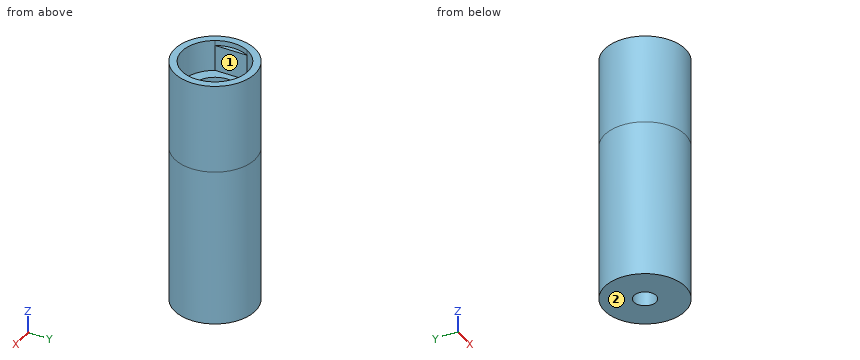
from build123d import *

# Parameters (mm, degrees)
F0_R     = 14.55
F1_DEPTH = 11.2
F2_DEPTH = 9.35
F0_R_2   = 7.975
F3_DEPTH = 21
F4_R     = 14.55
F4_R_2   = 4
F5_DEPTH = 57


with BuildPart() as f1:
    # F0 (on Top) → F1 (new body)
    with BuildSketch(Plane.XY):
        Circle(F0_R)
        with BuildLine():
            ThreePointArc((10.425, -5.7900777197), (0, -11.925), (-10.425, -5.7900777197))
            ThreePointArc((-10.425, -5.7900777197), (-11.925, 0), (-10.425, 5.7900777197))
            ThreePointArc((-10.425, 5.7900777197), (0, 11.925), (10.425, 5.7900777197))
            ThreePointArc((10.425, 5.7900777197), (11.925, 0), (10.425, -5.7900777197))
        make_face(mode=Mode.SUBTRACT)
    extrude(amount=F1_DEPTH)

    # F0 (on Top) → F2 (join)
    with BuildSketch(Plane.XY):
        with BuildLine():
            ThreePointArc((-10.425, 5.7900777197), (-11.925, 0), (-10.425, -5.7900777197))
            Line((-10.425, -5.7900777197), (-10.425, 5.7900777197))
        make_face()
        with BuildLine():
            Line((10.425, 5.7900777197), (10.425, -5.7900777197))
            ThreePointArc((10.425, -5.7900777197), (11.925, 0), (10.425, 5.7900777197))
        make_face()
    extrude(amount=F2_DEPTH)

    # F0 (on Top) → F3 (join)
    with BuildSketch(Plane.XY):
        Circle(F0_R)
        with BuildLine():
            ThreePointArc((10.425, -5.7900777197), (0, -11.925), (-10.425, -5.7900777197))
            ThreePointArc((-10.425, -5.7900777197), (-11.925, 0), (-10.425, 5.7900777197))
            ThreePointArc((-10.425, 5.7900777197), (0, 11.925), (10.425, 5.7900777197))
            ThreePointArc((10.425, 5.7900777197), (11.925, 0), (10.425, -5.7900777197))
        make_face(mode=Mode.SUBTRACT)
        with BuildLine():
            Line((-10.425, 5.7900777197), (-10.425, -5.7900777197))
            ThreePointArc((-10.425, -5.7900777197), (0, -11.925), (10.425, -5.7900777197))
            Line((10.425, -5.7900777197), (10.425, 5.7900777197))
            ThreePointArc((10.425, 5.7900777197), (0, 11.925), (-10.425, 5.7900777197))
        make_face()
        Circle(F0_R_2, mode=Mode.SUBTRACT)
        with BuildLine():
            Line((10.425, 5.7900777197), (10.425, -5.7900777197))
            ThreePointArc((10.425, -5.7900777197), (11.925, 0), (10.425, 5.7900777197))
        make_face()
        with BuildLine():
            ThreePointArc((-10.425, 5.7900777197), (-11.925, 0), (-10.425, -5.7900777197))
            Line((-10.425, -5.7900777197), (-10.425, 5.7900777197))
        make_face()
    extrude(amount=-F3_DEPTH)

    # F4 (on face) → F5 (join)
    with BuildSketch(Plane(origin=(0, 0, -21), x_dir=(1, 0, 0), z_dir=(0, 0, -1))):
        Circle(F4_R)
        Circle(F4_R_2, mode=Mode.SUBTRACT)
    extrude(amount=F5_DEPTH)


solid = f1.part
Design review of the part built by this model. Coordinates are the model's own, in mm. Face numbers are marked on the shaded views. Coordinates: 2 decimals unless noted, no trailing zeros. Loops run counter-clockwise (first coordinate to the right, second up) from the corner with the lowest first, then second, coordinate; pieces in that order, holes last. Notation, with made-up numbers: (8, 22) -> (47, 22) arc R14 ccw to (47, 33) -> close; hole circle Ø3 at (49.25, 44). An arc over 180 degrees is marked (long way). Use a Markdown table: item, result. Add a question column.
Item 1: We need section D-D, the plane y = 9.5. Write out the cut boundary in (x, z), and give its area (3 significant figures).
Item 2: We need section C-C, the plane z = -39. Write out the cut boundary in (x, y).
Item 3: Wall thickness on L1, parallel to X at y = 0, z = -65.5; L2, parallel to Y at x = 0, z = -9.75 (3 decimals): over which ranges is each line inside the solid? List them lowest first. Write a range as from..to.
Item 4: Clearance check with flat-ended pins moving along their axes: P1, Ø13, axis at x = -0.5, y = 3, coming from the +Z side; P2, Ø4.5, axis at y = 1, z = 6.5, coming from the +X side; P3, Ø1, axis at x = -4, z = -16, coming from the -Y side; P4, Ø4, axis at x = 8.5, y = 0, coming from the +Z side. State where each tip first meets the part, or that it passes through.
Item 5: The part is to be moulded in two halves that separate along Y. For the marked faces 1 and 2, say which applies: +Y half, -Y half, draft (parallel to the pull), parting line (faces both ways), or undercut.
Item 6: We need section B-B, the plane x = 0. Write out the cut boundary in (y, z) (3 decimals), and give its area (3 significant figures).
Item 7: We need section A-A, the plane y = 0. Write out the cut boundary in (x, z) (3 decimals).
Numbers:
| question | item | result |
|---|---|---|
| 1 | outline | (-11.02, -78) -> (11.02, -78) -> (11.02, 11.2) -> (7.21, 11.2) -> (7.21, 0) -> (-7.21, 0) -> (-7.21, 11.2) -> (-11.02, 11.2) -> close |
| 1 | area | 1,800 mm^2 |
| 2 | outline | circle Ø29.1 at (0, 0); hole circle Ø8 at (0, 0) |
| 3 | L1 | x = -14.55..-4, 4..14.55 |
| 3 | L2 | y = -14.55..-7.975, 7.975..14.55 |
| 4 | P1 | stops at z = 0 |
| 4 | P2 | stops at x = 14.55 |
| 4 | P3 | stops at y = -14.12 |
| 4 | P4 | stops at z = 9.35 |
| 5 | face 1 | undercut |
| 5 | face 2 | draft |
| 6 | outline | (-14.55, -78) -> (-4, -78) -> (-4, -21) -> (-7.975, -21) -> (-7.975, 0) -> (-11.925, 0) -> (-11.925, 11.2) -> (-14.55, 11.2) -> close; (4, -78) -> (14.55, -78) -> (14.55, 11.2) -> (11.925, 11.2) -> (11.925, 0) -> (7.975, 0) -> (7.975, -21) -> (4, -21) -> close |
| 6 | area | 1,540 mm^2 |
| 7 | outline | (-14.55, -78) -> (-4, -78) -> (-4, -21) -> (-7.975, -21) -> (-7.975, 0) -> (-10.425, 0) -> (-10.425, 9.35) -> (-11.925, 9.35) -> (-11.925, 11.2) -> (-14.55, 11.2) -> close; (4, -78) -> (14.55, -78) -> (14.55, 11.2) -> (11.925, 11.2) -> (11.925, 9.35) -> (10.425, 9.35) -> (10.425, 0) -> (7.975, 0) -> (7.975, -21) -> (4, -21) -> close |
